Autodesk Inventor part; units mm, degrees
ref_plane "YZ Plane" through (0, 0, 0) normal (1, 0, 0) x (0, 1, 0)
ref_plane "XZ Plane" through (0, 0, 0) normal (0, 1, 0) x (-1, 0, 0)
ref_plane "XY Plane" through (0, 0, 0) normal (0, 0, 1) x (1, 0, 0)
sketch "Sketch1" plane through (0, 0, 0) normal (0, 1, 0) x (-1, 0, 0)
  line L0 (-25, 225) -> (25, 225)
  line L1 (25, 225) -> (25, -225)
  line L2 (25, -225) -> (-25, -225)
  line L3 (-25, -225) -> (-25, 225)
  line L4 (-25, 225) -> (25, -225) construction
  line L5 (25, 225) -> (-25, -225) construction
  line L6 (0, 225) -> (0, 125)
  circle A0 centre (0, 125) radius 4
  line L7 (0, 125) -> (0, 50)
  circle A1 centre (0, 50) radius 4
  point P0 (0, 0)
  dimension "d0" = 50
  dimension "d1" = 450
  dimension "d6" = 100
  dimension "d7" = 8
  dimension "d8" = 75
  dimension "d9" = 8
extrude "Extrusion2" add sketch "Sketch1" along normal blind 2
properties part number "Lup"
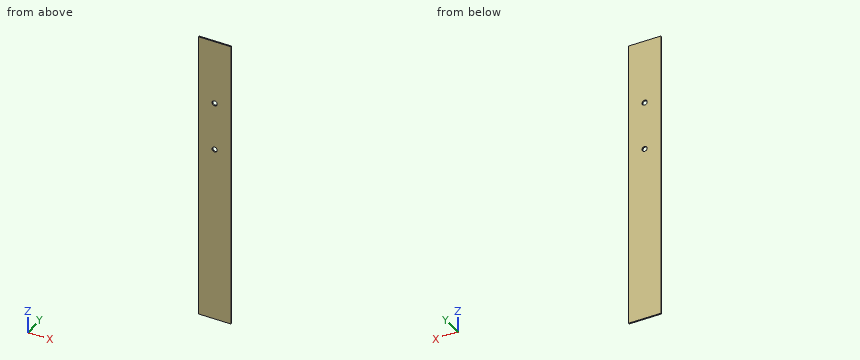
Verification items for the finished model (mm, model axes). Round coordinates to 2 decimals unless told otherwise and drop trailing zeros. Order: outer loops, then holes, each group sorted by start corner. A loop starts at its lowest first (then second) coordinate and runs counter-clockwise, first axis right, second up.
1. Section check B-B on z = 125. Record the cut outline in (x, y), then the cut area to 3 significant figures.
Final values:
outline: (-25, 0) - (-4, 0) - (-4, 2) - (-25, 2) - close; (4, 0) - (25, 0) - (25, 2) - (4, 2) - close
area: 84.0 mm2
2. Go/stop test with a flat-tipped pin: P1, Ø6.5, axis at x = 0, z = 125, coming from the -Y side. Record where the tip stops, or that it passes through.
Final values:
P1: passes through
3. Thickness scan on L1, parallel to Z at x = 0, y = 1.45; L2, parallel to Z at x = -3, y = 1.9; L3, parallel to X at y = 0.6, z = 50. Record the ranges inside material, lowest first.
Final values:
L1: z = -225 to 46, 54 to 121, 129 to 225
L2: z = -225 to 47.35, 52.65 to 122.35, 127.65 to 225
L3: x = -25 to -4, 4 to 25
4. Section check A-A on x = 0. Record the cut outline in (y, z), then the cut area to 3 significant figures.
Final values:
outline: (0, -225) - (2, -225) - (2, 46) - (0, 46) - close; (0, 54) - (2, 54) - (2, 121) - (0, 121) - close; (0, 129) - (2, 129) - (2, 225) - (0, 225) - close
area: 868 mm2
